Verification items for the finished model (mm, model axes). Give positions to 0.01 mm unless a question says otherwise; leave off trailing zeros. Order: outer loops, then holes, each group sorted by start corner. A loop starts at its lowest first (then second) coordinate and runs counter-clockwise, first axis right, second up. Notation, with made-up numbers: (-5, 4.5) -> (37, 4.5) arc R17 cw to (37, 26.5) -> close; hole circle Ø1 at (53, 34). An arc over 180 degrees is marked (long way). One line per question, with ' | ' between items. Start each with the question number.
Q1. Section check A-A on y = 0.15. Give the number of separate pieces and of enclosed holes in the cut face, plus the area to 3 significant figures.
Q2. Section check B-B on x = 14.7. Record the cut outline in (y, z), plus the area to 3 significant figures.
Q3. Section check D-D on x = 44. Record the cut outline in (y, z), plus the area to 3 significant figures.
Q4. Material ranges on probe 1 along Z at (x, y) = (69.6, 0.35); probe 2 along Z at (x, y) = (65, 0.35), recorded low to high. Write a range as [from, to].
Q5. Mould release check, pull along Z, two halves, no side actions. Record for faces 1 (the flat face through (43, 0, -2)), 2 (the cylindrical face through (18.91, 0.25, -1.71)): released by +Z, released by -Z, zero draft, split by the parting line, or undercut.
Q6. Go/stop test with a flat-tipped pin: pin 1 (3 mm diameter, centred on x = 69.5, z = -2, fed in from +Y). Record where the tip stops, or that it passes through.
Autodesk Inventor part; units mm, degrees
ref_plane "YZ Plane" through (0, 0, 0) normal (1, 0, 0) x (0, 1, 0)
ref_plane "XZ Plane" through (0, 0, 0) normal (0, 1, 0) x (-1, 0, 0)
ref_plane "XY Plane" through (0, 0, 0) normal (0, 0, 1) x (1, 0, 0)
sketch "Sketch1" plane through (0, 0, 0) normal (0, 1, 0) x (-1, 0, 0)
  line L0 (0, 0) -> (-84.3, 0)
  line L1 (-84.3, 0) -> (-84.3, -5)
  line L2 (-84.3, -5) -> (0, -5)
  line L3 (0, -5) -> (0, 0)
  circle A0 centre (-2.5, -2.5) radius 2.05
  circle A1 centre (-8.6, -2.5) radius 2.05
  circle A2 centre (-14.7, -2.5) radius 2.05
  circle A3 centre (-20.8, -2.5) radius 2.05
  circle A4 centre (-26.9, -2.5) radius 2.05
  circle A5 centre (-33, -2.5) radius 2.05
  circle A6 centre (-39.1, -2.5) radius 2.05
  circle A7 centre (-45.2, -2.5) radius 2.05
  circle A8 centre (-51.3, -2.5) radius 2.05
  circle A9 centre (-57.4, -2.5) radius 2.05
  circle A10 centre (-63.5, -2.5) radius 2.05
  circle A11 centre (-69.6, -2.5) radius 2.05
  circle A12 centre (-75.7, -2.5) radius 2.05
  circle A13 centre (-81.8, -2.5) radius 2.05
  dimension "d1" = 5
  dimension "d3" = 4.1
  dimension "d4" = 2.5
  dimension "d5" = 2.5
  dimension "d8" = 6.1
  dimension "d13" = 2.5
  dimension "d16" = 6.1
  dimension "d17" = 4.1
  dimension "d18" = 2.5
extrude "Extrusion1" add sketch "Sketch1" along normal blind 0.5
equation "\"d5\" = d4"
equation "\"d18\" = d5"
properties part number "separator-kul" material "Polycarbonate, Smoke"
Filled in:
1) separate pieces: 1 | enclosed holes: 14 | area: 237 mm²
2) outline: (0, -5) -> (0.5, -5) -> (0.5, -4.55) -> (0, -4.55) -> close; (0, -0.45) -> (0.5, -0.45) -> (0.5, 0) -> (0, 0) -> close | area: 0.450 mm²
3) outline: (0, -5) -> (0.5, -5) -> (0.5, -4.16) -> (0, -4.16) -> close; (0, -0.84) -> (0.5, -0.84) -> (0.5, 0) -> (0, 0) -> close | area: 0.838 mm²
4) probe 1: [-5, -4.55], [-0.45, 0] | probe 2: [-5, -3.9], [-1.1, 0]
5) face 1: zero draft | face 2: undercut
6) pin 1: through
